Autodesk Inventor part; units mm, degrees
ref_plane "YZ Plane" through (0, 0, 0) normal (1, 0, 0) x (0, 1, 0)
ref_plane "XZ Plane" through (0, 0, 0) normal (0, 1, 0) x (-1, 0, 0)
ref_plane "XY Plane" through (0, 0, 0) normal (0, 0, 1) x (1, 0, 0)
sketch "Sketch1" plane through (0, 0, 0) normal (0, 1, 0) x (-1, 0, 0)
  line L0 (0, 0) -> (25, 0)
  line L1 (25, 0) -> (25, -165)
  line L2 (25, -165) -> (0, -165)
  line L3 (0, -165) -> (0, 0)
  dimension "d0" = 25
  dimension "d1" = 165
extrude "Extrusion1" add sketch "Sketch1" along normal blind 3
sketch "Sketch2" plane through (0, 3, 0) normal (0, 1, 0) x (1, 0, 0)
  line L0 (-25, 165) -> (-25, 0)
  line L1 (0, 0) -> (0, 165)
  line L2 (-25, 0) -> (0, 0)
  line L3 (0, 0) -> (0, 7)
  line L4 (0, 7) -> (-25, 7)
  line L5 (-25, 7) -> (-25, 0)
  line L6 (0, 165) -> (-25, 165)
  line L7 (-25, 165) -> (0, 165)
  line L8 (0, 165) -> (0, 158)
  line L9 (0, 158) -> (-25, 158)
  line L10 (-25, 158) -> (-25, 165)
  dimension "d4" = 7
  dimension "d5" = 7
extrude "Extrusion2" add sketch "Sketch2" along normal blind 22 contours L6 L1 L9 L0 | L4 L1 L2 L0
sketch "Sketch3" plane through (-25, 0, 0) normal (0, 0, 1) x (1, 0, 0)
  point P0 (25, 0)
sketch "Sketch4" plane through (-25, 0, 0) normal (0, 0, 1) x (1, 0, 0)
  line L0 (25, 25) -> (0, 25) construction
  line L1 (25, 0) -> (0, 25) construction
  circle A0 centre (12.5, 12.5) radius 6.5
  dimension "d8" = 13
extrude "Extrusion3" cut sketch "Sketch4" against normal blind 5
sketch "Sketch5" plane through (0, 0, -165) normal (0, 0, -1) x (-1, 0, 0)
  circle A0 centre (12.5, 12.5) radius 6.5
  circle A1 centre (12.5, 12.5) radius 6.5
  point P0 (0, 0)
extrude "Extrusion4" cut sketch "Sketch5" against normal blind 5
sketch "Sketch6" plane through (-25, 0, 0) normal (0, 0, 1) x (1, 0, 0)
  circle A0 centre (12.5, 12.5) radius 6.5
  circle A1 centre (12.5, 12.5) radius 5
  point P0 (25, 0)
  dimension "d13" = 10
extrude "Extrusion5" cut sketch "Sketch6" against normal blind 165 contours A1
sketch "Sketch7" plane through (-25, 3, -158) normal (0, 0, 1) x (1, 0, 0)
  line L0 (25, 0) -> (25, 22) construction
  line L1 (0, 0) -> (0, 22) construction
  point P0 (25, -3)
sketch "Sketch8" plane through (-25, 3, -158) normal (0, 0, 1) x (1, 0, 0)
  circle A0 centre (12.5, 9.5) radius 5
  point P0 (25, -3)
sketch "Sketch9" plane through (0, 3, 0) normal (0, 1, 0) x (1, 0, 0)
  line L0 (-25, 158) -> (0, 158)
  line L1 (0, 7) -> (-25, 7)
  line L2 (-25, 158) -> (-20, 158)
  line L3 (-20, 158) -> (-20, 7)
  line L4 (-20, 7) -> (-25, 7)
  line L5 (-25, 7) -> (-25, 158)
  line L6 (0, 0) -> (0, 7)
  line L7 (0, 7) -> (-5, 7)
  line L8 (-5, 7) -> (-5, 158)
  line L9 (-5, 158) -> (0, 158)
  line L10 (0, 158) -> (0, 7)
  dimension "d16" = 5
  dimension "d17" = 5
extrude "Extrusion6" add sketch "Sketch9" along normal blind 7.5 contours L0 L3 L1 L5 | L0 L10 L1 L8
fillet "Fillet1" radius 2 2 edges at (-5, 10.5, -82.5) (-20, 10.5, -82.5)
sketch "Sketch10" plane through (0, 0, 0) normal (1, 0, 0) x (0, 0, -1)
  line L0 (0, 0) -> (0, 25)
  line L1 (165, 0) -> (0, 0)
  line L2 (0, 25) -> (16, 25)
  line L3 (16, 25) -> (16, 0)
  line L4 (16, 0) -> (0, 0)
  line L5 (0, 0) -> (0, 25)
  line L6 (165, 0) -> (165, 25)
  line L7 (165, 25) -> (149, 25)
  line L8 (149, 25) -> (149, 0)
  line L9 (149, 0) -> (165, 0)
  line L10 (165, 0) -> (165, 25)
  dimension "d21" = 16
  dimension "d22" = 16
extrude "Extrusion7" add sketch "Sketch10" along normal blind 45
sketch "Sketch11" plane through (45, 0, 0) normal (1, 0, 0) x (0, 0, -1)
  line L0 (7, 25) -> (0, 25) construction
  line L1 (16, 0) -> (16, 25) construction
  line L2 (0, 25) -> (16, 25) construction
  line L3 (16, 25) -> (7, 25) construction
  line L4 (8, 25) -> (8, 21.5) construction
  line L5 (14.125, 19.875) -> (1.875, 19.875)
  line L6 (1.875, 19.875) -> (1.875, 23.125)
  line L7 (1.875, 23.125) -> (14.125, 23.125)
  line L8 (14.125, 23.125) -> (14.125, 19.875)
  line L9 (14.125, 19.875) -> (1.875, 23.125) construction
  line L10 (1.875, 19.875) -> (14.125, 23.125) construction
  line L11 (165, 25) -> (149, 25) construction
  line L12 (157, 25) -> (157, 21.5) construction
  line L13 (163.125, 19.875) -> (150.875, 19.875)
  line L14 (150.875, 19.875) -> (150.875, 23.125)
  line L15 (150.875, 23.125) -> (163.125, 23.125)
  line L16 (163.125, 23.125) -> (163.125, 19.875)
  line L17 (163.125, 19.875) -> (150.875, 23.125) construction
  line L18 (150.875, 19.875) -> (163.125, 23.125) construction
  point P0 (0, 0)
  dimension "d25" = 3.5
  dimension "d26" = 12.25
  dimension "d27" = 3.25
  dimension "d28" = 3.5
  dimension "d29" = 12.25
  dimension "d30" = 3.25
extrude "Extrusion8" cut sketch "Sketch11" against normal blind 40
sketch "Sketch12" plane through (45, 0, 0) normal (1, 0, 0) x (0, 0, -1)
  line L0 (16, 0) -> (16, 25) construction
  line L1 (0, 19.875) -> (16, 19.875) construction
  line L2 (16, 19.875) -> (16, 18) construction
  line L3 (16, 18) -> (0, 18) construction
  line L4 (0, 18) -> (0, 19.875) construction
  point P0 (0, 0)
  dimension "d33" = 1.875
sketch "Sketch13" plane through (-25, 0, 0) normal (0, 0, 1) x (1, 0, 0)
  line L0 (70, 0) -> (70, 25) construction
  line L1 (70, 25) -> (70, 18) construction
  arc A0 (70, 18) -> (25, 0) centre (67.8851, -41.9627) ccw
  line L2 (70, 25) -> (70, 0)
  line L3 (70, 18) -> (70, 0)
  line L4 (70, 0) -> (25, 0)
  dimension "d34" = 7
  dimension "d35" = 60
extrude "Extrusion9" cut sketch "Sketch13" against normal blind 165
sketch "Sketch14" plane through (0, 10.5, 0) normal (0, 1, 0) x (1, 0, 0)
  point P0 (0, 0)
sketch "Sketch15" plane through (-25, 0, -165) normal (0, 0, -1) x (-1, 0, 0)
  circle A0 centre (-12.5, 12.5) radius 6.5 construction
  circle A1 centre (-12.5, 12.5) radius 25.4 construction
  point P0 (-25, 0)
  dimension "d38" = 50.8
sketch "Sketch16" plane through (0, 10.5, 0) normal (0, 1, 0) x (1, 0, 0)
  line L0 (-25, 0) -> (-25, 165)
  line L1 (-25, 82.5) -> (-32, 82.5)
  line L2 (-32, 82.5) -> (-32, 86)
  line L3 (-32, 86) -> (-25, 86)
  line L4 (-25, 86) -> (-25, 82.5)
  line L5 (-32, 82.5) -> (-25, 82.5)
  line L6 (-25, 82.5) -> (-25, 79)
  line L7 (-25, 79) -> (-32, 79)
  line L8 (-32, 79) -> (-32, 82.5)
  point P0 (0, 0)
  dimension "d39" = 7
  dimension "d40" = 3.5
  dimension "d41" = 3.5
extrude "Extrusion10" add sketch "Sketch16" against normal blind 10.5
sketch "Sketch17" plane through (0, 10.5, 0) normal (0, 1, 0) x (1, 0, 0)
  line L0 (-32, 79) -> (-25, 79) construction
  line L1 (-25, 86) -> (-32, 86) construction
  line L2 (-25, 79) -> (-32, 86) construction
  circle A0 centre (-28.5, 82.5) radius 3.175
  point P0 (0, 0)
  dimension "d44" = 6.35
extrude "Extrusion11" cut sketch "Sketch17" against normal blind 10.5
fillet "Fillet2" radius 7 2 edges at (-25, 5.25, -79) (-25, 5.25, -86)
sketch "Sketch18" plane through (0, 25, 0) normal (0, 1, 0) x (1, 0, 0)
  line L0 (45, 1.875) -> (45, 14.125) construction
  line L1 (45, 8) -> (20, 8) construction
  circle A0 centre (20, 8) radius 0.75
  line L2 (45, 150.875) -> (45, 163.125) construction
  line L3 (45, 157) -> (20, 157) construction
  circle A1 centre (20, 157) radius 0.75
  point P0 (0, 0)
  dimension "d48" = 25
  dimension "d49" = 1.5
  dimension "d50" = 25
  dimension "d51" = 1.5
extrude "Extrusion12" cut sketch "Sketch18" against normal blind 25
properties part number "frontAxelHolder 11-28"
For this review, take the finished solid that the model builds, in its own axes (mm). A direction names the side the tool comes from. Give positions to 0.01 mm unless a question says otherwise; leave off trailing zeros. Loops run counter-clockwise (first coordinate to the right, second up) from the corner with the lowest first, then second, coordinate; pieces in that order, holes last. Notation, with made-up numbers: M -4,60 L 39,60 A20 ccw 39,79 Z; hole C 16.5,-37.75 d5. An arc over 180 degrees is marked long. One line per item, written item: value. Start each with the question number.
Q1. For L1, parallel to Z at x = 20, y = 18; L2, parallel to Z at x = 4.5, y = 19.5; L3, parallel to Z at x = -23, y = 13, list the stretches that pass through material, from the lowest coordinate up.
Q2. Add section D-D (x = -28.5). Give the boundary of the cut face in (y, z) (3 decimals), and give its area (3 significant figures).
Q3. Add section A-A (x = -12.5). Give the boundary of the cut face in (y, z), and give its area (3 significant figures).
Q4. Machinability: for faces 4 (the face through (-25, 7, -128)), 5 (the face through (25, 23.125, -157)), 6 (the face through (0, 18, -153)), 7 (the face through (-10.6, 7.7, -5)), which of the approach directions +Z, -Z, +X, -X, +Y, -Y give a long, thin tool a straight path to every point of the face, cutting with its end or side? Answer none if there is none.
Q5. Clearance check with flat-ended pins moving along their axes: pin 1 Ø1.6 at (y, z) = (21.5, -160) entering from +X; pin 2 Ø16.5 at (x, z) = (-13.5, -66) entering from +Y; pin 3 Ø12 at (y, z) = (7.5, -123.5) entering from +X. State where each tip first meets the part, or that it passes through.
Q6. Add section B-B (z = -82.5). Give the boundary of the cut face in (x, y) (3 decimals), and give its area (3 significant figures).
Q7. Draft analysis for pull direction Y (two halves, no side actions). For faces 1 (the face through (45, 24, -157)), 2 (the face through (-12, 0, -81)), 3 (the face through (25, 23.125, -8)), state which applies: released by +Y, released by -Y, zero draft, split by the parting line, or undercut.
Q8. Add section C-C (z = -25.5). Give the boundary of the cut face in (x, y).
Reply:
1. L1: -165 to -157.75, -156.25 to -149, -16 to -8.75, -7.25 to 0
1. L2: -165 to -149, -16 to 0
1. L3: -165 to -158, -7 to 0
2. outline: M 0,-86.938 L 10.5,-86.938 L 10.5,-85.675 L 0,-85.675 Z; M 0,-79.325 L 10.5,-79.325 L 10.5,-78.062 L 0,-78.062 Z
2. area: 26.5 mm²
3. outline: M 0,-165 L 6,-165 L 6,-160 L 7.5,-160 L 7.5,-158 L 3,-158 L 3,-7 L 7.5,-7 L 7.5,-5 L 6,-5 L 6,0 L 0,0 Z; M 17.5,-160 L 19,-160 L 19,-165 L 25,-165 L 25,-158 L 17.5,-158 Z; M 17.5,-7 L 25,-7 L 25,0 L 19,0 L 19,-5 L 17.5,-5 Z
3. area: 633 mm²
4. face 4: -Z, -X, +Y, -Y
4. face 5: +X
4. face 6: -X, +Y
4. face 7: +Z
5. pin 1: x = 5
5. pin 2: y = 10.48
5. pin 3: x = 0
6. outline: M -32,0 L -31.675,0 L -31.675,10.5 L -32,10.5 Z; M -25.325,0 L 0,0 L 0,10.5 L -3,10.5 A2 ccw -5,8.5 L -5,3 L -20,3 L -20,8.5 A2 ccw -22,10.5 L -25.325,10.5 Z
6. area: 155 mm²
7. face 1: zero draft
7. face 2: released by -Y
7. face 3: undercut
8. outline: M -25,0 L 0,0 L 0,10.5 L -3,10.5 A2 ccw -5,8.5 L -5,3 L -20,3 L -20,8.5 A2 ccw -22,10.5 L -25,10.5 Z
